from build123d import *

# Parameters (mm, degrees)
EXTRUDE_1_DEPTH          = 100
CUT_EXTRUDE_START        = -2.5
CUT_EXTRUDE_1_OUTLINE_W  = 107.411770938
CUT_EXTRUDE_1_OUTLINE_H  = 17.637554046
CUT_EXTRUDE_1_OUTLINE_R  = 4
CUT_EXTRUDE_1_DEPTH      = 2.5
CUT_EXTRUDE_2_DEPTH      = 100
CUT_EXTRUDE_2_DEPTH_BACK = 100
SKETCH_6_W               = 1
SKETCH_6_H               = 5
M2X0_35_1_D              = 1.65
M2X0_35_1_DEPTH          = 2
M2X0_35_1_TIP            = 0.495710011


# Read off the part's stored shape, not the designer's step: 切除-拉伸1
with BuildPart() as part:
    # 草图1 → 凸台-拉伸1 (new body)
    with BuildSketch(Plane(origin=(0, 0, 0), x_dir=(0, 0, -1), z_dir=(1, 0, 0))):
        with BuildLine():
            Line((4.841229183, 1.25), (0, 1.25))
            Line((0, 1.25), (0, -1.25))
            Line((0, -1.25), (4.841229183, -1.25))
            ThreePointArc((4.841229183, -1.25), (4.960148481, -0.630021462), (5, 0))
            ThreePointArc((5, 0), (4.960148481, 0.630021462), (4.841229183, 1.25))
        make_face()
        with BuildLine():
            Line((0, -1.25), (0, 1.25))
            Line((0, 1.25), (-4.841229183, 1.25))
            ThreePointArc((-4.841229183, 1.25), (-5, 0), (-4.841229183, -1.25))
            Line((-4.841229183, -1.25), (0, -1.25))
        make_face()
    extrude(amount=EXTRUDE_1_DEPTH)

    # 切除-拉伸1 outline → 切除-拉伸1 (cut)
    # profile 1 of 3: a face of its own
    with BuildSketch(Plane(origin=(0, 1.25, 0), x_dir=(1, 0, 0), z_dir=(0, 1, 0)).offset(CUT_EXTRUDE_START)):
        with Locations((50.551661955, -0.114939413)):
            Rectangle(CUT_EXTRUDE_1_OUTLINE_W, CUT_EXTRUDE_1_OUTLINE_H)
        with BuildLine():
            Line((15.8786768, 5), (84.1213232, 5))
            ThreePointArc((84.1213232, 5), (89.1213232, 0), (84.1213232, -5))
            Line((84.1213232, -5), (15.8786768, -5))
            ThreePointArc((15.8786768, -5), (10.8786768, 0), (15.8786768, 5))
        make_face(mode=Mode.SUBTRACT)
    # profile 2 of 3: a face of its own
    with BuildSketch(Plane(origin=(0, 1.25, 0), x_dir=(1, 0, 0), z_dir=(0, 1, 0)).offset(CUT_EXTRUDE_START)):
        with BuildLine():
            Line((18.3786768, -1.658312395), (18.3786768, 1.658312395))
            ThreePointArc((18.3786768, 1.658312395), (12.8786768, 0), (18.3786768, -1.658312395))
        make_face()
    # profile 3 of 3: a face of its own
    with BuildSketch(Plane(origin=(0, 1.25, 0), x_dir=(1, 0, 0), z_dir=(0, 1, 0)).offset(CUT_EXTRUDE_START)):
        with Locations((84.1213232, 0)):
            Circle(CUT_EXTRUDE_1_OUTLINE_R)
    extrude(amount=CUT_EXTRUDE_1_DEPTH, mode=Mode.SUBTRACT)

    # 草图3 → 切除-旋转2 (revolve, cut)
    with BuildSketch(Plane(origin=(0, 0, 0), x_dir=(1, 0, 0), z_dir=(0, 1, 0))):
        with BuildLine():
            Line((12.414575185, -2), (10.590757267, -2))
            Line((10.590757267, -2), (10.590757267, -5))
            Line((10.590757267, -5), (84.1213232, -5))
            ThreePointArc((84.1213232, -5), (81.382710412, -4.183300133), (79.538747505, -2))
            Line((79.538747505, -2), (19.342778415, -2))
            ThreePointArc((19.342778415, -2), (15.8786768, -4), (12.414575185, -2))
        make_face()
        with BuildLine():
            Line((10.590757267, 5), (10.590757267, 2))
            Line((10.590757267, 2), (12.414575185, 2))
            ThreePointArc((12.414575185, 2), (15.8786768, 4), (19.342778415, 2))
            Line((19.342778415, 2), (79.538747505, 2))
            ThreePointArc((79.538747505, 2), (81.382710412, 4.183300133), (84.1213232, 5))
            Line((84.1213232, 5), (10.590757267, 5))
        make_face()
    revolve(axis=Axis((10.590757267, 0, 0), (1, 0, 0)), mode=Mode.SUBTRACT)

    # 草图6 → 切除-拉伸2 (cut, two sides: drawn at the far end of the back side and taken through both)
    with BuildSketch(Plane(origin=(0, 0, 0), x_dir=(1, 0, 0), z_dir=(0, 1, 0)).offset(-CUT_EXTRUDE_2_DEPTH_BACK)):
        with Locations((10.8786768, 0)):
            Rectangle(SKETCH_6_W, SKETCH_6_H)
    extrude(amount=CUT_EXTRUDE_2_DEPTH + CUT_EXTRUDE_2_DEPTH_BACK, mode=Mode.SUBTRACT)

    # M2X0.35 螺纹孔的螺纹孔钻头1
    with Locations(Plane.ZY.offset(-11.3786768)):
        with Locations((0, 0)):
            Hole(M2X0_35_1_D / 2, depth=M2X0_35_1_DEPTH)
            with Locations((0, 0, -(M2X0_35_1_DEPTH + M2X0_35_1_TIP / 2))):  # 118° drill point
                Cone(0, M2X0_35_1_D / 2, M2X0_35_1_TIP, mode=Mode.SUBTRACT)


solid = part.part
Could you check a few things on this model? Use its own coordinates, in mm. A direction names the side the tool comes from. Give positions to 0.01 mm unless a question says otherwise; leave off trailing zeros. Order: outer loops, then holes, each group sorted by start corner. A loop starts at its lowest first (then second) coordinate and runs counter-clockwise, first axis right, second up.
Item 1: If we section it at A-A, the plane z = 0: Write out the boundary of the cut face in (x, y) (3 decimals), plus the area to 3 significant figures.
Item 2: For faces 1 (the face through (18.379, 0, 0)), 2 (the face through (49, 0, 2)), 3 (the face through (12.198, 0.036, 0.824)), 4 (the face through (11.379, -1, 0)), 5 (the face through (49, 0, -2)), which set-ups out of +Z, -Z, +X, -X, +Y, -Y let a thin tool reach every point of the face, with its end or its side?
Item 3: I need wall thicknesses on line 1 (X direction, y = -0.95, z = 2.5); line 2 (X direction, y = -0.7, z = 0); line 3 (X direction, y = 0.5, z = -1.75). Which ranges of each line are inside material? Lowest first, please.
Item 4: I'm going to push flat-ended pins straight in: pin 1 (1.2 mm diameter, centred on y = 0, z = 0.5, fed in from -X); pin 2 (1 mm diameter, centred on x = 63.5, y = 0.5, fed in from +Z). Where does each tip first touch, or does it pass through?
Item 5: If we mould it in two halves opening along Z, with no side actions, what happens to faces 6 (the face through (47, 1.25, 0)), 7 (the face through (84.6, -0.78, -4.94)), 8 (the face through (80.125, -0.018, -0.176))? For each: pulls with the +Z half, pulls with the -Z half, needs draft (parallel to the pull), parting line crosses it, or undercut.
Item 6: If we section it at B-B, the plane x = 81: Write out the boundary of the cut face in (y, z).
Values:
1. outline: (11.379, -1.25) - (12.879, -1.25) - (12.879, -0.825) - (11.379, -0.825) - close; (11.379, 0.825) - (12.879, 0.825) - (12.879, 1.25) - (11.379, 1.25) - close; (18.379, -1.25) - (80.121, -1.25) - (80.121, 1.25) - (18.379, 1.25) - close; (88.121, -1.25) - (89.121, -1.25) - (89.121, 1.25) - (88.121, 1.25) - close
1. area: 158 mm2
2. face 1: +Y, -Y
2. face 2: +Z
2. face 3: -X
2. face 4: +Z, -Z, -X, +Y, -Y
2. face 5: -Z
3. line 1: x = 12.9 to 14.22, 17.54 to 18.85, 79.9 to 81, 87.24 to 88.45
3. line 2: x = 18.38 to 80.12, 88.12 to 89.12
3. line 3: x = 11.38 to 13.44, 18.32 to 80.52, 87.72 to 88.81
4. pin 1: stops at x = 11.38
4. pin 2: stops at z = 2
5. face 6: needs draft
5. face 7: pulls with the -Z half
5. face 8: undercut
6. outline: (-1.25, -3.7) arc R3.91 ccw to (1.25, -3.7) - (1.25, -2.5) - (-1.25, -2.5) - close; (-1.25, 2.5) - (1.25, 2.5) - (1.25, 3.7) arc R3.91 ccw to (-1.25, 3.7) - close
